Build history of the part. All positions in model axes, mm. Round coordinates to 2 decimals unless told otherwise and drop trailing zeros. Loops run counter-clockwise (first coordinate to the right, second up) from the corner with the lowest first, then second, coordinate; pieces in that order, holes last. Notation, with made-up numbers: (60, -6) - (81, -6) arc R25 ccw to (81, 17) - close; hole circle Ø6 at (80.25, 55.25). An arc over 180 degrees is marked (long way). Put each result on its own line as item: value. Start each with the question number.
from build123d import *

# Parameters (mm, degrees)
SKETCH_W     = 34.3
SKETCH_H     = 60.5
PAD_DEPTH    = 2.5
SKETCH001_W  = 2
SKETCH001_H  = 2
PAD001_DEPTH = 4


with BuildPart() as part:
    # Sketch → Pad (new body, symmetric)
    with BuildSketch(Plane.XY):
        Rectangle(SKETCH_W, SKETCH_H)
    extrude(amount=PAD_DEPTH, both=True)

    # Sketch001 → Pad001 (new body)
    with BuildSketch(Plane(origin=(0, 30.25, 0), x_dir=(-1, 0, 0), z_dir=(0, 1, 0))):
        with Locations((0, 1.5)):
            Rectangle(SKETCH001_W, SKETCH001_H)
    extrude(amount=PAD001_DEPTH)


solid = part.part
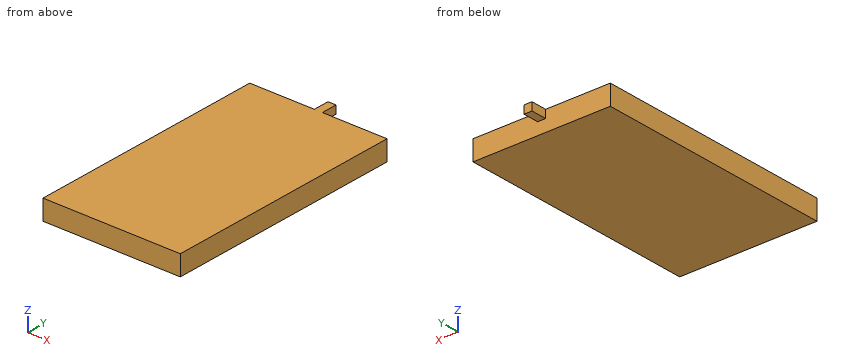
1) Slice it at A-A, the plane z = 1.7. Write the cut outline in (x, y).
2) Drill centre line: line 1 (Y direction, x = -2, z = 1.4). Where is it in solid material? Low to high. Write a range as [from, to].
3) Slice it at B-B, the plane x = 11.5. Write the cut outline in (y, z), and give its area (4 significant figures).
4) Drop flat-ended pins along their axis: pin 1 Ø2.5 at (x, z) = (7.5, 1) entering from +Y; pin 2 Ø1 at (y, z) = (31.5, 1.5) entering from +X; pin 3 Ø0.6 at (x, y) = (0.5, 31.5) entering from -Z. Give the stop position or say it passes through.
5) Slice it at C-C, the plane z = -1.5. Write the cut outline in (x, y).
Taken from the geometry:
1. outline: (-17.15, -30.25) - (17.15, -30.25) - (17.15, 30.25) - (1, 30.25) - (1, 34.25) - (-1, 34.25) - (-1, 30.25) - (-17.15, 30.25) - close
2. line 1: y = [-30.25, 30.25]
3. outline: (-30.25, -2.5) - (30.25, -2.5) - (30.25, 2.5) - (-30.25, 2.5) - close
3. area: 302.5 mm2
4. pin 1: stops at y = 30.25
4. pin 2: stops at x = 1
4. pin 3: stops at z = 0.5
5. outline: (-17.15, -30.25) - (17.15, -30.25) - (17.15, 30.25) - (-17.15, 30.25) - close
